from build123d import *

# Parameters (mm, degrees)
BOSS_EXTRUDE1_DEPTH = 463
SHELL2_T            = -2
SKETCH2_R           = 2.55
BOSS_EXTRUDE2_DEPTH = 2
SKETCH4_R           = 5.25
BOSS_EXTRUDE3_DEPTH = 2
BOSS_EXTRUDE4_DEPTH = 2
SKETCH6_R           = 38.1
CUT_EXTRUDE1_DEPTH  = 2


with BuildPart() as part:
    # Sketch1 → Boss-Extrude1 (new body)
    with BuildSketch(Plane.XY):
        with BuildLine():
            Line((-169.657845697, 59.751021298), (-110.243632135, 119.16523486))
            ThreePointArc((-110.243632135, 119.16523486), (-109.919208786, 119.382007611), (-109.536525354, 119.458128079))
            Line((-109.536525354, 119.458128079), (49.635047521, 119.458128079))
            ThreePointArc((49.635047521, 119.458128079), (50.017730954, 119.382007611), (50.342154303, 119.16523486))
            Line((50.342154303, 119.16523486), (109.756367865, 59.751021298))
            ThreePointArc((109.756367865, 59.751021298), (109.973140616, 59.426597949), (110.049261084, 59.043914516))
            Line((110.049261084, 59.043914516), (110.049261084, -80.540871921))
            ThreePointArc((110.049261084, -80.540871921), (110.048968191, -80.541579028), (110.048261084, -80.541871921))
            Line((110.048261084, -80.541871921), (-169.949738916, -80.541871921))
            ThreePointArc((-169.949738916, -80.541871921), (-169.950446023, -80.541579028), (-169.950738916, -80.540871921))
            Line((-169.950738916, -80.540871921), (-169.950738916, 59.043914516))
            ThreePointArc((-169.950738916, 59.043914516), (-169.874618449, 59.426597949), (-169.657845697, 59.751021298))
        make_face()
    extrude(amount=BOSS_EXTRUDE1_DEPTH)

    # Shell2
    shell2_openings = [part.faces().sort_by_distance(p)[0] for p in [
        (-29.950738916, 32.739133998, 463),
    ]]
    offset(amount=SHELL2_T, openings=shell2_openings, kind=Kind.INTERSECTION)

    # Sketch2 → Boss-Extrude2 (add)
    with BuildSketch(Plane(origin=(110.049261084, 0, 0), x_dir=(0, 0, -1), z_dir=(1, 0, 0))):
        with BuildLine():
            Line((-40, -80.540871921), (-9.025530914, -123.506525452))
            ThreePointArc((-9.025530914, -123.506525452), (-3.439175629, -125.291011633), (0, -120.540871921))
            Line((0, -120.540871921), (0, -80.540871921))
            Line((0, -80.540871921), (-40, -80.540871921))
        make_face()
        with Locations((-5, -120.540871921)):
            Circle(SKETCH2_R, mode=Mode.SUBTRACT)
    boss_extrude2 = extrude(amount=-BOSS_EXTRUDE2_DEPTH)

    # Mirror1: Boss-Extrude2 across plane
    add(boss_extrude2.mirror(Plane(origin=(-29.950738916, 0, 0), x_dir=(0, 0, 1), z_dir=(1, 0, 0))))

    # Sketch4 → Boss-Extrude3 (add)
    with BuildSketch(Plane(origin=(-49.950738916, 0, 0), x_dir=(0, 0, -1), z_dir=(1, 0, 0))):
        with BuildLine():
            Line((-352.326976552, -122.966309209), (-377.571249485, -80.540871921))
            Line((-377.571249485, -80.540871921), (-309.673952471, -80.540871921))
            Line((-309.673952471, -80.540871921), (-336.899509657, -123.589322478))
            ThreePointArc((-336.899509657, -123.589322478), (-344.793097516, -127.731489821), (-352.326976552, -122.966309209))
        make_face()
        with Locations((-344.43340661, -118.824585544)):
            Circle(SKETCH4_R, mode=Mode.SUBTRACT)
    boss_extrude3 = extrude(amount=-BOSS_EXTRUDE3_DEPTH)

    # Mirror2: Boss-Extrude3 across plane
    add(boss_extrude3.mirror(Plane(origin=(-29.950738916, 0, 0), x_dir=(0, 0, 1), z_dir=(1, 0, 0))))

    # Sketch5 → Boss-Extrude4 (add)
    with BuildSketch(Plane.XY.offset(463)):
        with BuildLine():
            Line((-165.021806728, 60.299996742), (-110.879671104, 114.442132366))
            ThreePointArc((-110.879671104, 114.442132366), (-107.635437616, 116.609859879), (-103.808603293, 117.371064554))
            Line((-103.808603293, 117.371064554), (48.049261084, 117.371064554))
            Line((48.049261084, 117.371064554), (105.120328896, 60.299996742))
            ThreePointArc((105.120328896, 60.299996742), (107.288056409, 57.055763254), (108.049261084, 53.22892893))
            Line((108.049261084, 53.22892893), (108.049261084, -78.541871921))
            Line((108.049261084, -78.541871921), (-167.950738916, -78.541871921))
            Line((-167.950738916, -78.541871921), (-167.950738916, 53.22892893))
            ThreePointArc((-167.950738916, 53.22892893), (-167.189534241, 57.055763254), (-165.021806728, 60.299996742))
        make_face()
    extrude(amount=-BOSS_EXTRUDE4_DEPTH)

    # Sketch6 → Cut-Extrude1 (cut)
    with BuildSketch(Plane.XY.offset(463)):
        with Locations((36.895099285, -27.454834831)):
            Circle(SKETCH6_R)
        with Locations((-96.144422598, -27.454834831)):
            Circle(SKETCH6_R)
        with Locations((-85.383873034, 62.216411536)):
            Circle(SKETCH6_R)
        with Locations((21.895545347, 62.216411536)):
            Circle(SKETCH6_R)
    extrude(amount=-CUT_EXTRUDE1_DEPTH, mode=Mode.SUBTRACT)


solid = part.part
Could you check a few things on this model? Use its own coordinates, in mm. A direction names the side the tool comes from. Coordinates: 2 decimals unless noted, no trailing zeros. Order: outer loops, then holes, each group sorted by start corner. A loop starts at its lowest first (then second) coordinate and runs counter-clockwise, first axis right, second up. Notation, with made-up numbers: (77, 55.25) - (87, 55.25) arc R11 ccw to (87, 65.25) - close; hole circle Ø2 at (21, 37.5). An arc over 180 degrees is marked (long way). Answer in a Markdown table with one row per item. Add a question column.
(1) If we section it at C-C, the plane y = -7: Please give me the cut outline in (x, z), then the cut area to 3 significant figures.
(2) If we mould it in two halves opening along X, with no side actions, what happens to faces 1 (the face through (108.049, -98, 16)), 2 (the face through (110.049, -11, 235)), 3 (the face through (-8.965, -101.764, 323.096))? For each: released by +X, released by -X, zero draft, split by the parting line, or undercut.
(3) If we section it at B-B, the plane x = -37.5: Please give me the cut outline in (y, z), then the cut area to 3 significant figures.
(4) On a 3-axis mill with a long thin cutter (end or side, diameter ignored), from which of +Z, -Z, +X, -X, +Y, -Y can I reach the whole of each face in a straight line? I mean faces 4 (the face through (-28, -78.542, 228)), 5 (the face through (-51.951, -99, 343)), 6 (the face through (73.236, -16.011, 462.014)), 7 (the face through (-8.965, -115.276, 348.303)), 8 (the face through (-7.951, -99, 343)). Say none if no direction works.
(5) If we section it at D-D, the plane x = 11: Please give me the cut outline in (y, z), then the cut area to 3 significant figures.
(6) I need wall thicknesses on L1, parallel to Y at x = -36, z = 435.5; L2, parallel to Z at x = 88, y = 21.5; L3, parallel to X at y = -18, z = 142. Which ranges of each line are inside material? Lowest first, please.
(7) Will these pins go through, and if not, where does the flat tip stop? pin 1 (23.5 mm diameter, centred on y = -95, z = 332, fed in from +X); pin 2 (6 mm diameter, centred on x = 34, z = 297, fed in from -Y); pin 3 (3 mm diameter, centred on x = -138, z = 382.5, fed in from +Y); pin 4 (4 mm diameter, centred on y = -120.54, z = 5, fed in from +X).
Results are:
| question | item | result |
|---|---|---|
| 1 | outline | (-169.95, 0) - (110.05, 0) - (110.05, 463) - (69.04, 463) - (69.04, 461) - (108.05, 461) - (108.05, 2) - (-167.95, 2) - (-167.95, 461) - (-128.29, 461) - (-128.29, 463) - (-169.95, 463) - close; (-64, 461) - (4.75, 461) - (4.75, 463) - (-64, 463) - close |
| 1 | area | 2,700 mm2 |
| 2 | face 1 | undercut |
| 2 | face 2 | released by +X |
| 2 | face 3 | zero draft |
| 3 | outline | (-80.54, 0) - (119.46, 0) - (119.46, 463) - (117.46, 463) - (117.46, 2) - (-78.54, 2) - (-78.54, 461) - (117.37, 461) - (117.37, 463) - (-80.54, 463) - close |
| 3 | area | 2,640 mm2 |
| 4 | face 4 | none |
| 4 | face 5 | +Z, -Z, -X, -Y |
| 4 | face 6 | +Z |
| 4 | face 7 | +X, -X |
| 4 | face 8 | +Z, -Z, +X, -Y |
| 5 | outline | (-80.54, 0) - (119.46, 0) - (119.46, 463) - (117.46, 463) - (117.46, 2) - (-78.54, 2) - (-78.54, 461) - (-55.4, 461) - (-55.4, 463) - (-80.54, 463) - close; (0.49, 461) - (25.71, 461) - (25.71, 463) - (0.49, 463) - close; (98.73, 461) - (117.37, 461) - (117.37, 463) - (98.73, 463) - close |
| 5 | area | 2,380 mm2 |
| 6 | L1 | y = -80.54 to -78.54, 117.46 to 119.46 |
| 6 | L2 | z = 0 to 2, 461 to 463 |
| 6 | L3 | x = -169.95 to -167.95, 108.05 to 110.05 |
| 7 | pin 1 | stops at x = -7.95 |
| 7 | pin 2 | stops at y = -80.54 |
| 7 | pin 3 | stops at y = 92.91 |
| 7 | pin 4 | passes through |
